Source: CAD feature listing. Evaluate the final solid. Frame: model axes, mm. Face numbers are marked on the shaded views. A direction names the side the tool comes from. Give positions to 0.01 mm unless a question says otherwise; leave off trailing zeros. Loops run counter-clockwise (first coordinate to the right, second up) from the corner with the lowest first, then second, coordinate; pieces in that order, holes last. Notation, with made-up numbers: (55.25, -25) -> (109.25, -25) arc R16 ccw to (109.25, -4) -> close; hole circle Ø1 at (19.5, 87.5). An arc over 180 degrees is marked (long way). Put each result on its own line as item: value.
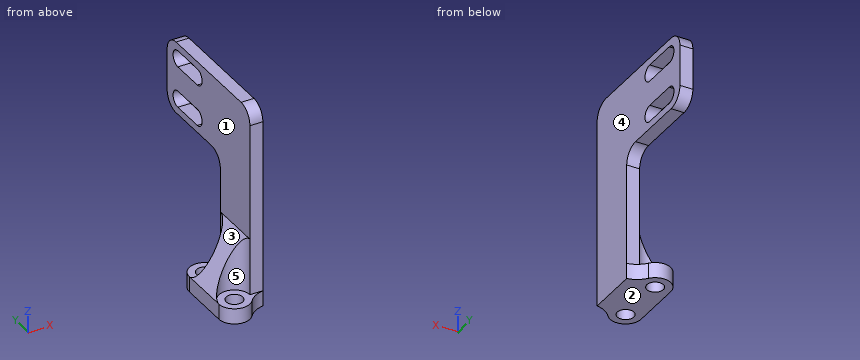
```python
from build123d import *

# Parameters (mm, degrees)
SKETCH_1_R          = 1.6
EXTRUDE_1_DEPTH     = 3
SKETCH_3_W          = 2.5
SKETCH_3_H          = 10
EXTRUDE_2_DEPTH     = 36.5
FILLET_1_R          = 5
FILLET_2_R          = 5
SKETCH_4_W          = 14
SKETCH_4_H          = 18
EXTRUDE_3_DEPTH     = 2.5
CUT_EXTRUDE_1_DEPTH = 62.232764559
EXTRUDE_4_DEPTH     = 10
SKETCH_8_R          = 3
CUT_EXTRUDE_2_DEPTH = 59.986875282
FILLET_3_R          = 3


with BuildPart() as part:
    # 草图1 → 凸台-拉伸1 (new body)
    with BuildSketch(Plane.XY):
        with BuildLine():
            ThreePointArc((3, -33.010340746), (0, -30.010340746), (-3, -33.010340746))
            Line((-3, -33.010340746), (-3, -43.010340746))
            ThreePointArc((-3, -43.010340746), (0, -46.010340746), (3, -43.010340746))
            Line((3, -43.010340746), (5.5, -43.010340746))
            Line((5.5, -43.010340746), (5.5, -33.010340746))
            Line((5.5, -33.010340746), (3, -33.010340746))
        make_face()
        with Locations((0, -33.010340746)):
            Circle(SKETCH_1_R, mode=Mode.SUBTRACT)
        with Locations((0, -43.010340746)):
            Circle(SKETCH_1_R, mode=Mode.SUBTRACT)
    extrude(amount=EXTRUDE_1_DEPTH)

    # 草图3 → 凸台-拉伸2 (add)
    with BuildSketch(Plane.XY.offset(3)):
        with Locations((4.25, -38.010340746)):
            Rectangle(SKETCH_3_W, SKETCH_3_H)
    extrude(amount=EXTRUDE_2_DEPTH)

    # 圆角1
    # the kernel refuses this fillet: 5 mm, written as the material it adds along each edge
    with BuildSketch(Plane(origin=(3, -43.010340746, 0), x_dir=(-0.32639560491693326, -0.9452332564456825, 0), z_dir=(0, 0, 1))) as fillet_1_piece_1:
        with BuildLine():
            CenterArc((3.590351654, 4.726166282), FILLET_1_R, 208.20428203, 42.745569225)
            Line((-0.815989012, 2.363083141), (0, 0))
            ThreePointArc((0, 0), (0.979186815, 0.164300231), (1.95837363, 0))
        make_face()
    extrude(amount=3)

    # 圆角2
    # the kernel refuses this fillet: 5 mm, written as the material it adds along each edge
    with BuildSketch(Plane(origin=(3, -33.010340746, 0), x_dir=(1, 0, 0), z_dir=(0, 0, 1))) as fillet_2_piece_1:
        with BuildLine():
            CenterArc((3.295454545, 4.936319688), FILLET_2_R, 218.100297491, 42.745569225)
            ThreePointArc((-0.639204545, 1.851119883), (-0.164300231, 0.979186815), (0, 0))
            Line((0, 0), (2.5, 0))
        make_face()
    extrude(amount=3)

    # 草图4 → 凸台-拉伸3 (add)
    with BuildSketch(Plane(origin=(5.5, 0, 0), x_dir=(0, 0, -1), z_dir=(1, 0, 0))):
        with Locations((-32.5, -24.010340746)):
            Rectangle(SKETCH_4_W, SKETCH_4_H)
    extrude(amount=-EXTRUDE_3_DEPTH)

    # 草图5 → 切除-拉伸1 (cut, through all)
    with BuildSketch(Plane(origin=(5.5, 0, 0), x_dir=(0, 0, -1), z_dir=(1, 0, 0))):
        with BuildLine():
            Line((-34.9, -18.617918523), (-34.9, -25.223242404))
            ThreePointArc((-34.9, -25.223242404), (-36.5, -26.823242404), (-38.1, -25.223242404))
            Line((-38.1, -25.223242404), (-38.1, -18.617918523))
            ThreePointArc((-38.1, -18.617918523), (-36.5, -17.017918523), (-34.9, -18.617918523))
        make_face()
        with BuildLine():
            Line((-30.1, -18.617918523), (-30.1, -25.223242404))
            ThreePointArc((-30.1, -25.223242404), (-28.5, -26.823242404), (-26.9, -25.223242404))
            Line((-26.9, -25.223242404), (-26.9, -18.617918523))
            ThreePointArc((-26.9, -18.617918523), (-28.5, -17.017918523), (-30.1, -18.617918523))
        make_face()
    extrude(amount=-CUT_EXTRUDE_1_DEPTH, mode=Mode.SUBTRACT)

    # 草图6 → 凸台-拉伸4 (add)
    with BuildSketch(Plane.XZ.offset(43.010340746)):
        Polygon((3, 14), (-3, 3), (3, 3), align=None)
    extrude(amount=-EXTRUDE_4_DEPTH)

    # 草图8 → 切除-拉伸2 (cut, through all)
    with BuildSketch(Plane.XY.offset(3)):
        with Locations((0, -43.010340746)):
            Circle(SKETCH_8_R)
        with Locations((0, -33.010340746)):
            Circle(SKETCH_8_R)
    extrude(amount=CUT_EXTRUDE_2_DEPTH, mode=Mode.SUBTRACT)

    # 圆角3
    fillet_3_edges = [part.edges().sort_by_distance(p)[0] for p in [
        (4.25, -43.010340746, 39.5),
        (4.25, -33.010340746, 25.5),
        (4.25, -15.010340746, 39.5),
        (4.25, -15.010340746, 25.5),
    ]]
    fillet(fillet_3_edges, radius=FILLET_3_R)


solid = part.part
```
(1) First-contact query: P1, Ø1.5, axis at x = 2, y = -33, coming from the +Z side; P2, Ø1.2, axis at x = 4, y = -22.5, coming from the -Z side; P3, Ø1.8, axis at x = 2, y = -41.5, coming from the +Z side. Flat tips, straight axial feed; report the tip coordinate or a pass-through.
Calculated:
P1: stops at z = 3
P2: stops at z = 25.5
P3: stops at z = 13.82
(2) Section B-B on y = -43.5. Return loops of the section in (x, z), then the cut area to 3 significant figures.
Calculated:
outline: (-2.96, 0) -> (-1.52, 0) -> (-1.52, 3) -> (-2.96, 3) -> close; (1.52, 0) -> (4.01, 0) -> (4.01, 3) -> (1.52, 3) -> close
area: 11.8 mm²
(3) Section C-C on y = -17.5. Return loops of the section in (x, z).
Calculated:
outline: (3, 25.54) -> (5.5, 25.54) -> (5.5, 27.36) -> (3, 27.36) -> close; (3, 29.64) -> (5.5, 29.64) -> (5.5, 35.36) -> (3, 35.36) -> close; (3, 37.64) -> (5.5, 37.64) -> (5.5, 39.46) -> (3, 39.46) -> close
(4) Section D-D on x = 3.5. Return loops of the section in (y, z), then the cut area to 3 significant figures.
Calculated:
outline: (-43.8, 0) -> (-32.22, 0) -> (-32.22, 3) -> (-33.01, 3) -> (-33.01, 22.5) arc R3 cw to (-30.01, 25.5) -> (-18.01, 25.5) arc R3 ccw to (-15.01, 28.5) -> (-15.01, 36.5) arc R3 ccw to (-18.01, 39.5) -> (-40.01, 39.5) arc R3 ccw to (-43.01, 36.5) -> (-43.01, 3) -> (-43.8, 3) -> close; hole (-25.22, 26.9) -> (-18.62, 26.9) arc R1.6 ccw to (-18.62, 30.1) -> (-25.22, 30.1) arc R1.6 ccw to start; hole (-25.22, 34.9) -> (-18.62, 34.9) arc R1.6 ccw to (-18.62, 38.1) -> (-25.22, 38.1) arc R1.6 ccw to start
area: 590 mm²
(5) Draft query along X for the marked faces 3, 4 and 5. Return one class per face: released by +X, released by -X, zero draft, split by the parting line, or undercut.
Calculated:
face 3: released by -X
face 4: released by +X
face 5: undercut
(6) Section A-A on x = 0. Return loops of the section in (y, z), then the cut area to 3 significant figures.
Calculated:
outline: (-46.01, 0) -> (-44.61, 0) -> (-44.61, 3) -> (-46.01, 3) -> close; (-41.41, 0) -> (-34.61, 0) -> (-34.61, 3) -> (-36.01, 3) -> (-36.01, 8.5) -> (-40.01, 8.5) -> (-40.01, 3) -> (-41.41, 3) -> close; (-31.41, 0) -> (-30.01, 0) -> (-30.01, 3) -> (-31.41, 3) -> close
area: 50.8 mm²
(7) Reachability of the marked faces 1 and 2 from +Z, -Z, +X, -X, +Y, -Y: full face, straight path, thin tool, end or side. Return the list, or none.
Calculated:
face 1: +Z, -X, +Y, -Y
face 2: -Z, +X, -X, +Y, -Y
(8) Line query: probe 1 along Z at (x, y) = (4.5, -20); probe 2 along Y at (x, z) = (0, 1.3); probe 3 along Z at (x, y) = (4, -18). Output: solid intervals per line, ascending. Write a range as from..to.
Calculated:
probe 1: z = 25.5..26.9, 30.1..34.9, 38.1..39.5
probe 2: y = -46.01..-44.61, -41.41..-34.61, -31.41..-30.01
probe 3: z = 25.5..27.02, 29.98..35.02, 37.98..39.5
